```python
from build123d import *

# Parameters (mm, degrees)
F0_R     = 7.5
F1_DEPTH = 3
F0_R_2   = 5.5
F2_DEPTH = 5
F3_ANGLE = 270


with BuildPart() as f1:
    # F0 (on Top) → F1 (new body)
    with BuildSketch(Plane.XY):
        with BuildLine():
            Line((100, 9.5), (0, 9.5))
            ThreePointArc((0, 9.5), (-6.717514, 6.717514), (-9.5, 0))
            ThreePointArc((-9.5, 0), (-6.717514, -6.717514), (0, -9.5))
            Line((0, -9.5), (100, -9.5))
            ThreePointArc((100, -9.5), (106.717514, -6.717514), (109.5, 0))
            ThreePointArc((109.5, 0), (106.717514, 6.717514), (100, 9.5))
        make_face()
        Circle(F0_R, mode=Mode.SUBTRACT)
        with Locations((20, 0)):
            Circle(F0_R, mode=Mode.SUBTRACT)
        with Locations((40, 0)):
            Circle(F0_R, mode=Mode.SUBTRACT)
        with Locations((60, 0)):
            Circle(F0_R, mode=Mode.SUBTRACT)
        with Locations((80, 0)):
            Circle(F0_R, mode=Mode.SUBTRACT)
        with Locations((100, 0)):
            Circle(F0_R, mode=Mode.SUBTRACT)
    extrude(amount=F1_DEPTH)

    # F0 (on Top) → F2 (join)
    with BuildSketch(Plane.XY):
        Circle(F0_R)
        Circle(F0_R_2, mode=Mode.SUBTRACT)
        with Locations((20, 0)):
            Circle(F0_R)
        with Locations((20, 0)):
            Circle(F0_R_2, mode=Mode.SUBTRACT)
        with Locations((40, 0)):
            Circle(F0_R)
        with Locations((40, 0)):
            Circle(F0_R_2, mode=Mode.SUBTRACT)
        with Locations((60, 0)):
            Circle(F0_R)
        with Locations((60, 0)):
            Circle(F0_R_2, mode=Mode.SUBTRACT)
        with Locations((80, 0)):
            Circle(F0_R)
        with Locations((80, 0)):
            Circle(F0_R_2, mode=Mode.SUBTRACT)
        with Locations((100, 0)):
            Circle(F0_R)
        with Locations((100, 0)):
            Circle(F0_R_2, mode=Mode.SUBTRACT)
    extrude(amount=F2_DEPTH)


with BuildPart() as f3_1:
    # F3: copy of F1
    add(f1.part.rotate(Axis((0, 0, 0), (0, 0, -1)), F3_ANGLE))


with BuildPart() as f3_1_1:
    # F4: moved
    add(f3_1.part.moved(Location((20, 0, 0))))


solid = f1.part
```
Build history of the part. All positions in model axes, mm. A direction names the side the tool comes from. Give positions to 0.01 mm unless a question says otherwise; leave off trailing zeros. Loops run counter-clockwise (first coordinate to the right, second up) from the corner with the lowest first, then second, coordinate; pieces in that order, holes last. Notation, with made-up numbers: (29.25, 82.25) - (78.25, 82.25) arc R10 cw to (78.25, 94.25) - close; hole circle Ø7 at (77.5, 81). An arc over 180 degrees is marked (long way). Use a Markdown table: item, result.
(1) Band-saw the part on B-B (z = 2.2). Give the cut face in (x, y), and give its area (3 significant figures).
Taken from the geometry:
| item | result |
|---|---|
| outline | (-9.5, 0) arc R9.5 ccw to (0, -9.5) - (100, -9.5) arc R9.5 ccw to (109.5, 0) arc R9.5 ccw to (100, 9.5) - (0, 9.5) arc R9.5 ccw to start; hole circle Ø11 at (0, 0); hole circle Ø11 at (20, 0); hole circle Ø11 at (40, 0); hole circle Ø11 at (60, 0); hole circle Ø11 at (80, 0); hole circle Ø11 at (100, 0) |
| area | 1,610 mm2 |
(2) Drop flat-ended pins along their axis: pin 1 Ø6 at (x, y) = (21, 0.5) entering from -Z; pin 2 Ø1 at (y, z) = (5.5, 3) entering from -X. Give the stop position or say it passes through.
Taken from the geometry:
| item | result |
|---|---|
| pin 1 | through |
| pin 2 | x = -8.08 |
(3) Band-saw the part on D-D (x = 31). Give the cut face in (y, z), and give its area (3 significant figures).
Taken from the geometry:
| item | result |
|---|---|
| outline | (-9.5, 0) - (9.5, 0) - (9.5, 3) - (-9.5, 3) - close |
| area | 57.0 mm2 |
(4) Which spindle directions (+Z, -Z, +X, -X, +Y, -Y) get a long thin tool onto all of the face, cutting with end or side? Do faces 1 (the face through (92.507, 0.33, 3.986)), 2 (the face through (49, 0, 0)). Say none if no direction does.
Taken from the geometry:
| item | result |
|---|---|
| face 1 | +Z |
| face 2 | -Z, +X, -X, +Y, -Y |
(5) Wall check: line 1 along Y through (x, z) = (80, 2.45); line 2 along Y through (x, z) = (100, 3.8); line 3 along Z through (x, y) = (92, -1.75). Give the ranges that are in metal, low to high.
Taken from the geometry:
| item | result |
|---|---|
| line 1 | -9.5 to -5.5, 5.5 to 9.5 |
| line 2 | -7.5 to -5.5, 5.5 to 7.5 |
| line 3 | 0 to 3 |
(6) Band-saw the part on C-C (y = 6.5). Give the cut face in (x, z), and give its area (3 significant figures).
Taken from the geometry:
| item | result |
|---|---|
| outline | (-6.93, 0) - (106.93, 0) - (106.93, 3) - (103.74, 3) - (103.74, 5) - (96.26, 5) - (96.26, 3) - (83.74, 3) - (83.74, 5) - (76.26, 5) - (76.26, 3) - (63.74, 3) - (63.74, 5) - (56.26, 5) - (56.26, 3) - (43.74, 3) - (43.74, 5) - (36.26, 5) - (36.26, 3) - (23.74, 3) - (23.74, 5) - (16.26, 5) - (16.26, 3) - (3.74, 3) - (3.74, 5) - (-3.74, 5) - (-3.74, 3) - (-6.93, 3) - close |
| area | 431 mm2 |
(7) Pull direction X, two halves, no side cores. Call faces 3 (the face through (51, 9.5, 1)), 4 (the face through (-1.19, -5.37, 2.46)): +X half, -X half, draft (parallel to the pull), parting line (faces both ways), or undercut.
Taken from the geometry:
| item | result |
|---|---|
| face 3 | draft |
| face 4 | undercut |
(8) Band-saw the part on A-A (x = 80). Give the cut face in (y, z).
Taken from the geometry:
| item | result |
|---|---|
| outline | (-9.5, 0) - (-5.5, 0) - (-5.5, 5) - (-7.5, 5) - (-7.5, 3) - (-9.5, 3) - close; (5.5, 0) - (9.5, 0) - (9.5, 3) - (7.5, 3) - (7.5, 5) - (5.5, 5) - close |
